Could you check a few things on this model? Use its own coordinates, in mm. A direction names the side the tool comes from. Coordinates: 2 decimals unless noted, no trailing zeros. Order: outer loops, then holes, each group sorted by start corner. A loop starts at its lowest first (then second) coordinate and runs counter-clockwise, first axis right, second up. Notation, with made-up numbers: (34.25, 54) - (63.25, 54) arc R25 ccw to (63.25, 85) - close; hole circle Ø3 at (60, 85). An arc over 180 degrees is marked (long way). Answer as a JSON object with one key per item and string values. Group by question number.
(1) We'd pull the mould along Y, two halves only. Please class faces 1 (the flat face through (32, 39.68, 1)), 2 (the cylindrical face through (29.775, -1.242, 1.479)), 3 (the cylindrical face through (41.827, 0.162, 1.479)), 4 (the cylindrical face through (39.57, 1.38, 1.48)): pulls with the +Y half, pulls with the -Y half, needs draft (parallel to the pull), parting line crosses it, or undercut.
(2) Which directions (+Z, -Z, +X, -X, +Y, -Y) give clear straight access to the entire face, cutting with the end or side of a thin tool? Please do faces 5 (the flat face through (33, 18, 0)), 6 (the cylindrical face through (38.26, 4.04, 1.48)).
(3) Imagine slicing it at B-B, the plane z = 0.95. Write out the boundary of the cut face in (x, y), and give its area (3 significant figures).
(4) Imagine slicing it at C-C, the plane x = 29.75. Write out the boundary of the cut face in (y, z).
(5) Imagine slicing it at D-D, the plane y = 23.5. Write out the boundary of the cut face in (x, z).
(6) Will this pin go through, and if not, where does the flat tip stop? P1, Ø1, axis at y = 8.5, z = 2.5, coming from the +X side.
(7) Imagine slicing it at A-A, the plane x = 39. Write out the boundary of the cut face in (y, z), and give its area (3 significant figures).
(8) Please list where these lines run through material, in increasing order: probe 1 along Y at (x, z) = (39.75, 2.6); probe 2 along Y at (x, z) = (40, 2.1); probe 3 along X at (y, z) = (37.5, 2).
from build123d import *

# Parameters (mm, degrees)
SALIENTE_EXTRUIR1_DEPTH = 3


with BuildPart() as part:
    # Model → Saliente-Extruir1 (new body)
    with BuildSketch(Plane.XY):
        with BuildLine():
            Line((27.467941077, 39.680349578), (27.467941077, 22.097099578))
            Line((27.467941077, 22.097099578), (27.467941077, 3.513849578))
            ThreePointArc((27.467941077, 3.513849578), (29.833805345, -1.291965393), (34.967941077, -2.819650422))
            ThreePointArc((34.967941077, -2.819650422), (37.2653644, -3.903815719), (39.800359504, -4.069248896))
            ThreePointArc((39.800359504, -4.069248896), (40.5704791, -3.527774359), (40.549576341, -2.586582592))
            ThreePointArc((40.549576341, -2.586582592), (39.682712456, -1.563786177), (38.497352842, -0.937297481))
            ThreePointArc((38.497352842, -0.937297481), (39.816352512, -1.009870934), (41.116644878, -0.776918583))
            ThreePointArc((41.116644878, -0.776918583), (41.8274431, 0.180349578), (41.116644878, 1.137617739))
            ThreePointArc((41.116644878, 1.137617739), (39.545301969, 1.380701786), (37.967941077, 1.180349578))
            ThreePointArc((37.967941077, 1.180349578), (39.230469791, 1.72740936), (40.379023795, 2.485087958))
            ThreePointArc((40.379023795, 2.485087958), (40.687813038, 3.636299223), (39.675412289, 4.265332526))
            ThreePointArc((39.675412289, 4.265332526), (38.236782457, 4.035665244), (36.849346326, 3.591341219))
            ThreePointArc((36.849346326, 3.591341219), (36.009082944, 3.632037192), (35.497205789, 4.299630249))
            ThreePointArc((35.497205789, 4.299630249), (35.415004717, 4.995458697), (35.476051331, 5.693461244))
            Line((35.476051331, 5.693461244), (35.493981077, 29.680349578))
            Line((35.493981077, 29.680349578), (35.493981077, 39.680349578))
            Line((35.493981077, 39.680349578), (27.467941077, 39.680349578))
        make_face()
    extrude(amount=SALIENTE_EXTRUIR1_DEPTH)


solid = part.part
Result set:
{
 "1": {"face 1": "pulls with the +Y half", "face 2": "pulls with the -Y half", "face 3": "parting line crosses it", "face 4": "undercut"},
 "2": {"face 5": "-Z, +X, -X, +Y, -Y", "face 6": "+Z, -Z, +Y"},
 "3": {"outline": "(27.47, 3.51) arc R6.69 ccw to (34.97, -2.82) arc R6.8 ccw to (39.8, -4.07) arc R1 ccw to (40.55, -2.59) arc R3.54 ccw to (38.5, -0.94) arc R5.7 ccw to (41.12, -0.78) arc R1 ccw to (41.12, 1.14) arc R5.7 ccw to (37.97, 1.18) arc R7.91 ccw to (40.38, 2.49) arc R1 ccw to (39.68, 4.27) arc R9.62 ccw to (36.85, 3.59) arc R1 cw to (35.5, 4.3) arc R3.43 cw to (35.48, 5.69) - (35.49, 29.68) - (35.49, 39.68) - (27.47, 39.68) - close", "area": "371 mm^2"},
 "4": {"outline": "(-1.22, 0) - (39.68, 0) - (39.68, 3) - (-1.22, 3) - close"},
 "5": {"outline": "(27.47, 0) - (35.49, 0) - (35.49, 3) - (27.47, 3) - close"},
 "6": {"P1": "stops at x = 35.48"},
 "7": {"outline": "(-4.12, 0) - (-1.13, 0) - (-1.13, 3) - (-4.12, 3) - close; (-1, 0) - (1.36, 0) - (1.36, 3) - (-1, 3) - close; (1.61, 0) - (4.19, 0) - (4.19, 3) - (1.61, 3) - close", "area": "23.8 mm^2"},
 "8": {"probe 1": "y = -4.08 to -1.62, -1.01 to 1.37, 2.03 to 4.27", "probe 2": "y = -4.02 to -1.85, -1 to 1.36, 2.2 to 4.24", "probe 3": "x = 27.47 to 35.49"}
}
